The model under review builds one solid part; all positions refer to its coordinate system, in mm. Face numbers are marked on the shaded views. A direction names the side the tool comes from. Coordinates: 2 decimals unless noted, no trailing zeros. Write each loop counter-clockwise with the first axis right and the second up, starting at its lowest first coordinate (ties: lowest second). Pieces come first, ordered by that corner, then holes. Notation, with made-up numbers: M -39.75,15.25 L -13.75,15.25 A9 cw -13.75,31.25 Z; hole C -16,6 d10. An arc over 180 degrees is marked long. Answer as a JSON object with one key per item and string values.
Autodesk Inventor part; units mm, degrees
ref_plane "YZ Plane" through (0, 0, 0) normal (1, 0, 0) x (0, 1, 0)
ref_plane "XZ Plane" through (0, 0, 0) normal (0, 1, 0) x (-1, 0, 0)
ref_plane "XY Plane" through (0, 0, 0) normal (0, 0, 1) x (1, 0, 0)
sketch "Szkic1" plane through (0, 0, 0) normal (0, 0, 1) x (1, 0, 0)
  circle A0 centre (-8.8768, 43) radius 2
  circle A1 centre (8.8768, 43) radius 2
  circle A2 centre (0, 27.625) radius 2
  line L0 (20.7693, 46.5287) -> (55.6245, -37.125)
  arc A3 (20.7693, 46.5287) -> (-20.7693, 46.5287) centre (0, 37.875) ccw
  line L1 (-55.6245, -37.125) -> (-20.7693, 46.5287)
  line L2 (-55.6245, -63.375) -> (-55.6245, -37.125)
  line L3 (55.6245, -63.375) -> (-55.6245, -63.375)
  line L4 (55.6245, -37.125) -> (55.6245, -63.375)
  circle A4 centre (-50, -53.375) radius 2.75
  circle A5 centre (50, -53.375) radius 2.75
  circle A6 centre (-25, -45.375) radius 2.75
  circle A7 centre (25, -45.375) radius 2.75
  circle A8 centre (0, -53.375) radius 2.75
  circle A9 centre (0, 37.875) radius 17.2375
  circle A10 centre (0, 37.875) radius 2.1667
  point P0 (0, 0)
extrude "Wyciągnięcie proste1" add sketch "Szkic1" along normal blind 2.54 contours A9
sketch "Szkic2" plane through (0, 37.875, 2.54) normal (0, 0, 1) x (1, 0, 0)
  circle A0 centre (0, 0) radius 17.2375
  circle A1 centre (0, 0) radius 2.1667
  circle A2 centre (0, -10.25) radius 2
  circle A3 centre (8.8768, 5.125) radius 2
  circle A4 centre (-8.8768, 5.125) radius 2
  point P0 (0, -37.875)
extrude "Wyciągnięcie proste2" cut sketch "Szkic2" against normal blind 0.54
sketch "Szkic3" plane through (0, 37.875, 2) normal (0, 0, 1) x (1, 0, 0)
  circle A0 centre (0, 0) radius 17.2375
  circle A1 centre (-8.8768, 5.125) radius 2
  circle A2 centre (8.8768, 5.125) radius 2
  circle A3 centre (0, -10.25) radius 2
  circle A4 centre (0, 0) radius 2.1667
  point P0 (0, -37.875)
extrude "Wyciągnięcie proste3" add sketch "Szkic3" against normal up to surface (2 mm away) contours A4
sketch "Szkic4" plane through (0, 37.875, 2) normal (0, 0, 1) x (1, 0, 0)
  circle A0 centre (0, 0) radius 17.2375
  circle A1 centre (-8.8768, 5.125) radius 2
  circle A2 centre (8.8768, 5.125) radius 2
  circle A3 centre (0, -10.25) radius 2
  circle A4 centre (0, 0) radius 2.15
  line L0 (2.15, 0) -> (4.15, 0)
  circle A5 centre (0, 0) radius 4.15
  point P0 (0, -37.875)
  dimension "d6" = 4.3
  dimension "d7" = 2
extrude "Wyciągnięcie proste4" add sketch "Szkic4" along normal blind 5 contours A5
sketch "Szkic5" plane through (0, 37.875, 2) normal (0, 0, 1) x (1, 0, 0)
  circle A0 centre (0, 0) radius 2.15
  point P0 (0, -37.875)
extrude "Wyciągnięcie proste5" add sketch "Szkic5" along normal blind 3
sketch "Szkic6" plane through (0, 37.875, 2) normal (0, 0, 1) x (1, 0, 0)
  circle A0 centre (0, 0) radius 17.2375
  circle A1 centre (-8.8768, 5.125) radius 2
  circle A2 centre (8.8768, 5.125) radius 2
  circle A3 centre (0, -10.25) radius 2
  circle A4 centre (0, -10.25) radius 2.25
  circle A5 centre (-8.8768, 5.125) radius 2.25
  circle A6 centre (8.8768, 5.125) radius 2.25
  point P0 (0, -37.875)
  dimension "d16" = 4.5
  dimension "d17" = 4.5
  dimension "d18" = 4.5
extrude "Wyciągnięcie proste6" cut sketch "Szkic6" against normal through all contours A1 | A2 | A3 | A4 | A5 | A6
properties part number "na magnes"
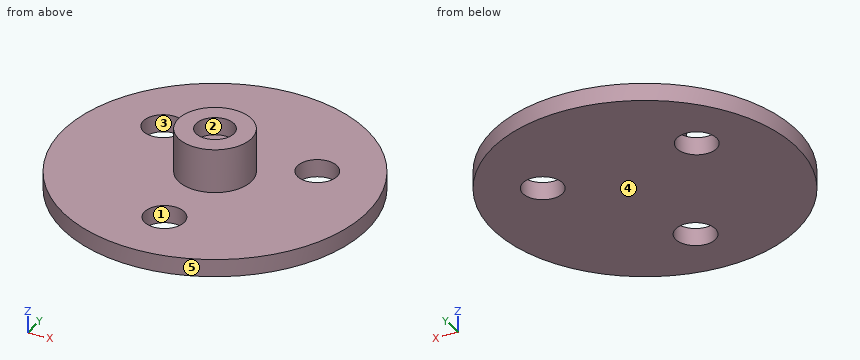
(1) Add section C-C on z = 3.5. Give the boundary of the cut face in (x, y) (3 decimals), and give its area (3 significant figures).
Results list:
{"outline": "C 0,37.875 d8.3", "area": "54.1 mm²"}
(2) Add section A-A on x = 0. Give the boundary of the cut face in (y, z) (1 decimal), and give its area (4 significant figures).
Results list:
{"outline": "M 20.6,0 L 25.4,0 L 25.4,2 L 20.6,2 Z; M 29.9,0 L 55.1,0 L 55.1,2 L 42,2 L 42,7 L 40,7 L 40,5 L 35.7,5 L 35.7,7 L 33.7,7 L 33.7,2 L 29.9,2 Z", "area": "92.85 mm²"}
(3) For pin 1 Ø3 at (x, z) = (-1.5, 6) entering from -Y (3 decimals); pin 2 Ø3 at (y, z) = (37.5, 5) entering from -X; pin 3 Ø1.5 at (x, z) = (5.5, 1.5) entering from -Y, all flat-tipped, find the tip position at first contact; note any pin that passes through.
Results list:
{"pin 1": "y = 33.725", "pin 2": "x = -4.15", "pin 3": "y = 21.3"}
(4) Wall thickness on line 1 along Y through (x, z) = (0, 0.55) (1 decimal); line 2 along Y through (x, z) = (0, 5.75) (3 decimals); line 3 along Z through (x, y) = (11.5, 40.5): over which ranges is each line inside the solid? List them lowest first. Write a range as from..to.
Results list:
{"line 1": "20.6..25.4, 29.9..55.1", "line 2": "33.725..35.725, 40.025..42.025", "line 3": "0..2"}
(5) Add section D-D on y = 50.5. Give the boundary of the cut face in (x, z).
Results list:
{"outline": "M -11.74,0 L 11.74,0 L 11.74,2 L -11.74,2 Z"}
(6) For the marked faces 1 and 2, list the 3-axis set-ups (+Z, -Z, +X, -X, +Y, -Y) from which the entire face can be reached by the end or side of a thin tool; tool diameter is ignored.
Results list:
{"face 1": "+Z, -Z", "face 2": "+Z"}
(7) Add section B-B on y = 43. Give the boundary of the cut face in (x, z).
Results list:
{"outline": "M -16.46,0 L -11.13,0 L -11.13,2 L -16.46,2 Z; M -6.63,0 L 6.63,0 L 6.63,2 L -6.63,2 Z; M 11.13,0 L 16.46,0 L 16.46,2 L 11.13,2 Z"}
(8) Draft analysis for pull direction X (two halves, no side actions). For the marked faces 3, 4 and 5, state which applies: released by +X, released by -X, zero draft, split by the parting line, or undercut.
Results list:
{"face 3": "undercut", "face 4": "zero draft", "face 5": "split by the parting line"}
